```python
from build123d import *

# Parameters (mm, degrees)
MAIN_EXTRUDE_ANGLE = 60
SKETCH4_R          = 3.175
SPAR_HOLES_1_DEPTH = 12.7
SKETCH5_R          = 3.175
SPAR_HOLES_2_DEPTH = 12.7


with BuildPart() as part:
    # Sketch3 → Main extrude (revolve)
    with BuildSketch(Plane.XY):
        with BuildLine():
            ThreePointArc((-2.267771894, 148.348367024), (0, 149.744334404), (2.267771894, 148.348367024))
            add(Edge.make_bspline(
                [(2.267771894, 148.348367024), (30.572440123, 92.24111101), (0, -152.4)],
                knots=[0, 0, 0, 1, 1, 1], degree=2))
            add(Edge.make_bspline(
                [(-2.267771894, 148.348367024), (-30.572440123, 92.24111101), (0, -152.4)],
                knots=[0, 0, 0, 1, 1, 1], degree=2))
        make_face()
        with BuildLine():
            Line((3.81, 57.15), (3.81, -6.35))
            ThreePointArc((3.81, -6.35), (0, -10.16), (-3.81, -6.35))
            Line((-3.81, -6.35), (-3.81, 57.15))
            ThreePointArc((-3.81, 57.15), (0, 60.96), (3.81, 57.15))
        make_face(mode=Mode.SUBTRACT)
    revolve(axis=Axis((-25.4, 132.199806754, 0), (0, -1, 0)), revolution_arc=MAIN_EXTRUDE_ANGLE)

    # Sketch4 → Spar holes 1 (cut)
    with BuildSketch(Plane(origin=(-19.05, 0, 10.998522628), x_dir=(0.5, 0, 0.866025404), z_dir=(-0.866025404, 0, 0.5))):
        with Locations((12.7, 82.55)):
            Circle(SKETCH4_R)
        with Locations((12.7, -31.75)):
            Circle(SKETCH4_R)
    extrude(amount=-SPAR_HOLES_1_DEPTH, mode=Mode.SUBTRACT)

    # Sketch5 → Spar holes 2 (cut)
    with BuildSketch(Plane(origin=(0, 0, 0), x_dir=(-1, 0, 0), z_dir=(0, 0, -1))):
        with Locations((0, 82.55)):
            Circle(SKETCH5_R)
        with Locations((0, -31.75)):
            Circle(SKETCH5_R)
    extrude(amount=-SPAR_HOLES_2_DEPTH, mode=Mode.SUBTRACT)


solid = part.part
```
Geometry: final body of the model. Coordinates: model frame, mm. A direction names the side the tool comes from. Give positions to 0.01 mm unless a question says otherwise; leave off trailing zeros. Answer as CSV lines item,"result". Start each with the question number.
1) First-contact query: P1, Ø1.9, axis at x = -1, y = 83, coming from the -Z side; P2, Ø10, axis at x = 0, y = 82.55, coming from the +Z side; P3, Ø6, axis at y = -23.5, z = 28, coming from the +X side. Flat tips, straight axial feed; report the tip coordinate or a pass-through.
2) Set-up query: faces 4 (the cylindrical face through (0.69, -34.85, 6.26)), 5 (the flat face through (-1.724, -31.706, 15.609)). Return all of +Z, -Z, +X, -X, +Y, -Y with unobstructed straight access to the full face (end or side cutting, diameter ignored); none if empty.
3) Line query: line 1 (X direction, y = -31, z = 3); line 2 (X direction, y = 31.5, z = 11); line 3 (Z direction, x = -1, y = 116). Output: solid intervals per line, ascending. Write a range as from..to.
4) Mould query, pull axis X, two halves, no side actions, for faces 1 (the flat face through (9, 11, 0)), 2 (the flat face through (-8.099, 10.568, 29.965)), 3 (the flat face through (0, 83, 12.7)). Classes: +X half, -X half, draft (parallel to the pull), parting line (faces both ways), or undercut.
Findings below:
1,P1,"stops at z = 12.7"
1,P2,"stops at z = 34.97"
1,P3,"stops at x = 3.74"
2,face 4,"-Z"
2,face 5,"none"
3,line 1,"x = -12.8..-3.09, 3.09..12.33"
3,line 2,"x = -19.05..-6.82, 1.66..14.14"
3,line 3,"z = 0..27.86"
4,face 1,"draft"
4,face 2,"-X half"
4,face 3,"undercut"
